```python
from build123d import *

# Parameters (mm, degrees)
SKETCH1_R           = 1.7
BOSS_EXTRUDE1_DEPTH = 100
SKETCH2_R           = 24.727322232
BOSS_EXTRUDE2_DEPTH = 10
FILLET2_R           = 3


with BuildPart() as part:
    # Sketch1 → Boss-Extrude1 (new body)
    with BuildSketch(Plane.XY):
        Circle(SKETCH1_R)
    extrude(amount=BOSS_EXTRUDE1_DEPTH)

    # Sketch2 → Boss-Extrude2 (add)
    with BuildSketch(Plane.XY.offset(100)):
        Circle(SKETCH2_R)
    extrude(amount=BOSS_EXTRUDE2_DEPTH)

    # Fillet2
    fillet2_edges = [part.edges().sort_by_distance(p)[0] for p in [
        (-1.7, 0, 100),
        (-24.727322232, 0, 100),
        (-24.727322232, 0, 110),
    ]]
    fillet(fillet2_edges, radius=FILLET2_R)


solid = part.part
```
Check sheet for the modelled part. Datum: model origin and axes. Units: mm. A direction names the side the tool comes from. Give positions to 0.01 mm unless a question says otherwise; leave off trailing zeros. Order: outer loops, then holes, each group sorted by start corner. A loop starts at its lowest first (then second) coordinate and runs counter-clockwise, first axis right, second up. Notation, with made-up numbers: M 17.25,76 L 55.25,76 A27 ccw 55.25,103 Z; hole C 33,20 d4. An arc over 180 degrees is marked long. Answer in a Markdown table with one row per item. Add a question column.
Q1. Thickness scan on L1, parallel to Z at x = 20.5, y = -3; L2, parallel to Z at x = 14.5, y = -17; L3, parallel to X at y = 1.5, z = 35.5. Record the ranges inside material, lowest first.
Q2. Gauge pin test, flat ends, axial feed: pin 1 Ø3 at (x, y) = (19.5, 0) entering from -Z; pin 2 Ø10 at (y, z) = (-2.5, 17.5) entering from -X; pin 3 Ø3 at (y, z) = (0, 87.5) entering from +X. Record the tip position at first contact, or that the pin passes through.
Q3. Access from +Z, -Z, +X, -X, +Y, -Y to the whole of each face (thin tool, end or side, straight path). Record for faces 1 (the flat face through (0, 0, 110)), 2 (the cylindrical face through (-0.37, -1.66, 47.82)).
Q4. Sectioned sample at A-A, the plane x = 0. Record the boundary of the cut face in (y, z).
Q5. Sectioned sample at C-C, the plane z = 61.5. Record the boundary of the cut face in (x, y), and give its area (3 significant figures).
Verdict:
| question | item | result |
|---|---|---|
| 1 | L1 | 100 to 110 |
| 1 | L2 | 100.06 to 109.94 |
| 1 | L3 | -0.8 to 0.8 |
| 2 | pin 1 | z = 100 |
| 2 | pin 2 | x = -1.7 |
| 2 | pin 3 | x = 1.7 |
| 3 | face 1 | +Z, +X, -X, +Y, -Y |
| 3 | face 2 | -Z |
| 4 | outline | M -24.73,103 A3 ccw -21.73,100 L -4.7,100 A3 cw -1.7,97 L -1.7,0 L 1.7,0 L 1.7,97 A3 cw 4.7,100 L 21.73,100 A3 ccw 24.73,103 L 24.73,107 A3 ccw 21.73,110 L -21.73,110 A3 ccw -24.73,107 Z |
| 5 | outline | C 0,0 d3.4 |
| 5 | area | 9.08 mm² |
